from build123d import *

# Parameters (mm, degrees)
SKETCH_1_W          = 15
SKETCH_1_H          = 15
SKETCH_1_W_2        = 13
SKETCH_1_H_2        = 13
EXTRUDE_1_DEPTH     = 570
SKETCH_2_R          = 1.45
CUT_EXTRUDE_1_DEPTH = 571.246657158
SKETCH_3_R          = 1.45
CUT_EXTRUDE_2_DEPTH = 571.246657158


with BuildPart() as part:
    # 草图1 → 凸台-拉伸1 (new body)
    with BuildSketch(Plane(origin=(0, 0, 0), x_dir=(0, 0, -1), z_dir=(1, 0, 0))):
        Rectangle(SKETCH_1_W, SKETCH_1_H)
        Rectangle(SKETCH_1_W_2, SKETCH_1_H_2, mode=Mode.SUBTRACT)
    extrude(amount=EXTRUDE_1_DEPTH)

    # 草图2 → 切除-拉伸1 (cut, through all)
    with BuildSketch(Plane(origin=(0, 7.5, 0), x_dir=(1, 0, 0), z_dir=(0, 1, 0))):
        with Locations(Location((566, 0, 0), (0, 0, 270))):
            Circle(SKETCH_2_R)
        with Locations(Location((556, 0, 0), (0, 0, 270))):
            Circle(SKETCH_2_R)
        with Locations(Location((485, 0, 0), (0, 0, 270))):
            Circle(SKETCH_2_R)
        with Locations(Location((460, 0, 0), (0, 0, 270))):
            Circle(SKETCH_2_R)
        with Locations(Location((297.5, 0, 0), (0, 0, 270))):
            Circle(SKETCH_2_R)
        with Locations(Location((272.5, 0, 0), (0, 0, 270))):
            Circle(SKETCH_2_R)
        with Locations(Location((110, 0, 0), (0, 0, 270))):
            Circle(SKETCH_2_R)
        with Locations(Location((85, 0, 0), (0, 0, 270))):
            Circle(SKETCH_2_R)
        with Locations(Location((14, 0, 0), (0, 0, 270))):
            Circle(SKETCH_2_R)
        with Locations(Location((4, 0, 0), (0, 0, 270))):
            Circle(SKETCH_2_R)
        with Locations(Location((512.5, 0, 0), (0, 0, 270))):
            Circle(SKETCH_2_R)
        with Locations(Location((57.5, 0, 0), (0, 0, 270))):
            Circle(SKETCH_2_R)
        with Locations(Location((504, 0, 0), (0, 0, 270))):
            Circle(SKETCH_2_R)
        with Locations(Location((537, 0, 0), (0, 0, 270))):
            Circle(SKETCH_2_R)
        with Locations(Location((66, 0, 0), (0, 0, 270))):
            Circle(SKETCH_2_R)
        with Locations(Location((33, 0, 0), (0, 0, 270))):
            Circle(SKETCH_2_R)
        with Locations(Location((225, 0, 0), (0, 0, 270))):
            Circle(SKETCH_2_R)
        with Locations(Location((346.5, 0, 0), (0, 0, 270))):
            Circle(SKETCH_2_R)
        with Locations(Location((326.5, 0, 0), (0, 0, 270))):
            Circle(SKETCH_2_R)
        with Locations(Location((248.5, 0, 0), (0, 0, 270))):
            Circle(SKETCH_2_R)
        with Locations(Location((184, 0, 0), (0, 0, 270))):
            Circle(SKETCH_2_R)
        with Locations(Location((194, 0, 0), (0, 0, 270))):
            Circle(SKETCH_2_R)
        with Locations(Location((376, 0, 0), (0, 0, 270))):
            Circle(SKETCH_2_R)
        with Locations(Location((386, 0, 0), (0, 0, 270))):
            Circle(SKETCH_2_R)
    extrude(amount=-CUT_EXTRUDE_1_DEPTH, mode=Mode.SUBTRACT)

    # 草图3 → 切除-拉伸2 (cut, through all)
    with BuildSketch(Plane(origin=(0, 0, -7.5), x_dir=(-1, 0, 0), z_dir=(0, 0, -1))):
        with Locations((-130, 0)):
            Circle(SKETCH_3_R)
        with Locations((-165, 0)):
            Circle(SKETCH_3_R)
        with Locations((-405, 0)):
            Circle(SKETCH_3_R)
        with Locations((-440, 0)):
            Circle(SKETCH_3_R)
    extrude(amount=-CUT_EXTRUDE_2_DEPTH, mode=Mode.SUBTRACT)


solid = part.part
The listing builds one solid part. Answer for the finished solid, in the listing's coordinates (mm). A direction names the side the tool comes from. Coordinates: 2 decimals unless noted, no trailing zeros. Order: outer loops, then holes, each group sorted by start corner. A loop starts at its lowest first (then second) coordinate and runs counter-clockwise, first axis right, second up. Notation, with made-up numbers: M 17.25,87 L 24.25,87 A30 cw 24.25,113 Z; hole C 13.5,74.25 d7. An arc over 180 degrees is marked long. Use CSV: the item, a comma, the result in double quotes.
Q1. Section A-A (y = -3.75) is taken. Determine the outline of the cut face in (x, z).
Here are the results:
outline,"M 0,-7.5 L 570,-7.5 L 570,-6.5 L 0,-6.5 Z; M 0,6.5 L 570,6.5 L 570,7.5 L 0,7.5 Z"
Q2. Straight lines are drawn through the part: L1, parallel to Y at x = 370, z = 3.25; L2, parallel to Y at x = 165, z = -6.85. For each, find the intervals that lie inside material, in ascending order.
Here are the results:
L1,"-7.5 to -6.5, 6.5 to 7.5"
L2,"-7.5 to -1.45, 1.45 to 7.5"
Q3. A tool of negligible diameter and unlimited length cuts with its end or side. For faces 1 (the flat face through (570, 0, 7)), 2 (the flat face through (281, 0, 6.5)), from which of +Z, -Z, +X, -X, +Y, -Y can it reach the whole face along a straight path? Write none if from no direction.
Here are the results:
face 1,"+Z, -Z, +X, +Y, -Y"
face 2,"+X, -X"
Q4. Determine the mould class of faces 3 (the flat face through (281, -6.5, 0)), 4 (the flat face through (281, 0, 7.5)), 5 (the flat face through (281, -7.5, 0)) for opening direction Z: pulls with the +Z half, pulls with the -Z half, needs draft (parallel to the pull), parting line crosses it, or undercut.
Here are the results:
face 3,"undercut"
face 4,"pulls with the +Z half"
face 5,"needs draft"
